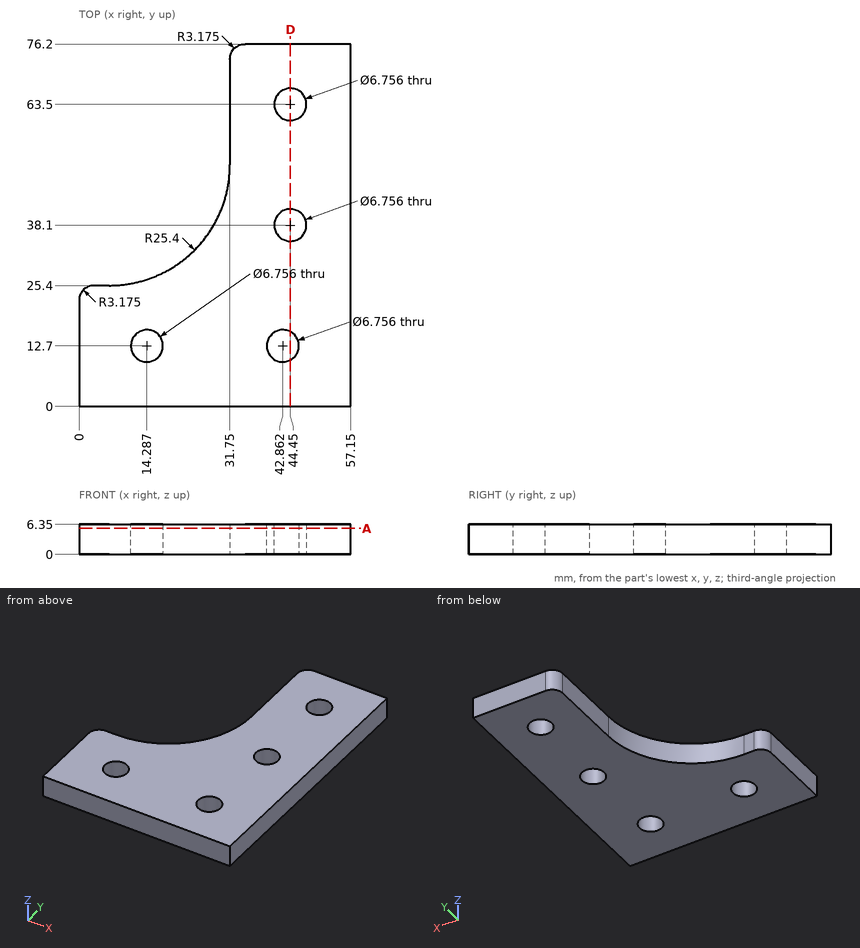
Check sheet for the drawn part. Datum: minimum x, y, z corner. Units: mm. Coordinates: 2 decimals unless noted, no trailing zeros. Write each loop counter-clockwise with the first axis right and the second up, starting at its lowest first coordinate (ties: lowest second). Pieces come first, ordered by that corner, then holes. Notation, with made-up numbers: M 30,78.5 L 79,78.5 A27 ccw 79,109.5 Z; hole C -2,68.25 d6. An arc over 180 degrees is marked long. One line per item, written item: value.
Item 1: Section check D-D, the plane x = 44.45. Record the boundary of the cut face in (y, z), plus the area to 3 significant figures.
Check sheet entries:
outline: M 0,0 L 9.72,0 L 9.72,6.35 L 0,6.35 Z; M 15.68,0 L 34.72,0 L 34.72,6.35 L 15.68,6.35 Z; M 41.48,0 L 60.12,0 L 60.12,6.35 L 41.48,6.35 Z; M 66.88,0 L 76.2,0 L 76.2,6.35 L 66.88,6.35 Z
area: 360 mm^2
Item 2: Gauge pin test, flat ends, axial feed: pin 1 Ø1 at (x, z) = (4.5, 3) entering from +Y; pin 2 Ø4 at (x, y) = (44.45, 63.5) entering from -Z; pin 3 Ø3 at (y, z) = (58.5, 3) entering from -X. Record the tip position at first contact, or that the pin passes through.
Check sheet entries:
pin 1: stops at y = 25.4
pin 2: passes through
pin 3: stops at x = 31.75
Item 3: Scan lines: line 1 along Y through (x, z) = (44.45, 3); line 2 along Y through (x, z) = (5.5, 4.75); line 3 along Y through (x, z) = (18.5, 2.25) (1 decimal). Record each from-to range of solid material in increasing order.
Check sheet entries:
line 1: y = 0 to 9.72, 15.68 to 34.72, 41.48 to 60.12, 66.88 to 76.2
line 2: y = 0 to 25.4
line 3: y = 0 to 28.5
Item 4: Section check A-A, the plane z = 5.5. State how many separate pieces and enclosed holes the cut face has, plus the area to 3 significant figures.
Check sheet entries:
separate pieces: 1
enclosed holes: 4
area: 2,730 mm^2
